```python
from build123d import *

# Parameters (mm, degrees)
F0_R     = 10.5
F0_R_2   = 6
F1_DEPTH = 15
F2_R     = 9
F2_R_2   = 6
F3_DEPTH = 10
F5_DEPTH = 4
F6_SIZE  = 0.5
F7_SIZE  = 0.5


with BuildPart() as f1:
    # F0 (on Top) → F1 (new body)
    with BuildSketch(Plane.XY):
        Circle(F0_R)
        Circle(F0_R_2, mode=Mode.SUBTRACT)
    extrude(amount=F1_DEPTH)

    # F2 (on face) → F3 (cut)
    with BuildSketch(Plane.XY.offset(15)):
        Circle(F2_R)
        Circle(F2_R_2, mode=Mode.SUBTRACT)
    extrude(amount=-F3_DEPTH, mode=Mode.SUBTRACT)

    # F4 (on face) → F5 (cut)
    with BuildSketch(Plane(origin=(0, 0, 0), x_dir=(1, 0, 0), z_dir=(0, 0, -1))):
        with BuildLine():
            Line((1.25, 8.25), (1.25, 13))
            Line((1.25, 13), (-1.25, 13))
            Line((-1.25, 13), (-1.25, 8.25))
            ThreePointArc((-1.25, 8.25), (-1.1767766953, 8.0732233047), (-1, 8))
            Line((-1, 8), (1, 8))
            ThreePointArc((1, 8), (1.1767766953, 8.0732233047), (1.25, 8.25))
        make_face()
        with BuildLine():
            Line((-6.5197095812, 5.2075317547), (-10.6333302492, 7.5825317547))
            Line((-10.6333302492, 7.5825317547), (-11.8833302492, 5.4174682453))
            Line((-11.8833302492, 5.4174682453), (-7.7697095812, 3.0424682453))
            ThreePointArc((-7.7697095812, 3.0424682453), (-7.5800048199, 3.0174931396), (-7.4282032303, 3.1339745962))
            Line((-7.4282032303, 3.1339745962), (-6.4282032303, 4.8660254038))
            ThreePointArc((-6.4282032303, 4.8660254038), (-6.4032281246, 5.0557301651), (-6.5197095812, 5.2075317547))
        make_face()
        with BuildLine():
            Line((-7.7697095812, -3.0424682453), (-11.8833302492, -5.4174682453))
            Line((-11.8833302492, -5.4174682453), (-10.6333302492, -7.5825317547))
            Line((-10.6333302492, -7.5825317547), (-6.5197095812, -5.2075317547))
            ThreePointArc((-6.5197095812, -5.2075317547), (-6.4032281246, -5.0557301651), (-6.4282032303, -4.8660254038))
            Line((-6.4282032303, -4.8660254038), (-7.4282032303, -3.1339745962))
            ThreePointArc((-7.4282032303, -3.1339745962), (-7.5800048199, -3.0174931396), (-7.7697095812, -3.0424682453))
        make_face()
        with BuildLine():
            Line((-1.25, -8.25), (-1.25, -13))
            Line((-1.25, -13), (1.25, -13))
            Line((1.25, -13), (1.25, -8.25))
            ThreePointArc((1.25, -8.25), (1.1767766953, -8.0732233047), (1, -8))
            Line((1, -8), (-1, -8))
            ThreePointArc((-1, -8), (-1.1767766953, -8.0732233047), (-1.25, -8.25))
        make_face()
        with BuildLine():
            Line((6.5197095812, -5.2075317547), (10.6333302492, -7.5825317547))
            Line((10.6333302492, -7.5825317547), (11.8833302492, -5.4174682453))
            Line((11.8833302492, -5.4174682453), (7.7697095812, -3.0424682453))
            ThreePointArc((7.7697095812, -3.0424682453), (7.5800048199, -3.0174931396), (7.4282032303, -3.1339745962))
            Line((7.4282032303, -3.1339745962), (6.4282032303, -4.8660254038))
            ThreePointArc((6.4282032303, -4.8660254038), (6.4032281246, -5.0557301651), (6.5197095812, -5.2075317547))
        make_face()
        with BuildLine():
            Line((7.7697095812, 3.0424682453), (11.8833302492, 5.4174682453))
            Line((11.8833302492, 5.4174682453), (10.6333302492, 7.5825317547))
            Line((10.6333302492, 7.5825317547), (6.5197095812, 5.2075317547))
            ThreePointArc((6.5197095812, 5.2075317547), (6.4032281246, 5.0557301651), (6.4282032303, 4.8660254038))
            Line((6.4282032303, 4.8660254038), (7.4282032303, 3.1339745962))
            ThreePointArc((7.4282032303, 3.1339745962), (7.5800048199, 3.0174931396), (7.7697095812, 3.0424682453))
        make_face()
    extrude(amount=-F5_DEPTH, mode=Mode.SUBTRACT)

    # F6
    f6_edges = [f1.edges().sort_by_distance(p)[0] for p in [
        (-5.25, -9.093267, 0),
        (5.25, -9.093267, 0),
        (10.286224, 2.107984, 0),
        (5.25, 9.093267, 0),
        (-5.25, 9.093267, 0),
        (-10.5, 0, 0),
    ]]
    chamfer(f6_edges, length=F6_SIZE)

    # F7
    f7_edges = [f1.edges().sort_by_distance(p)[0] for p in [
        (-10.5, 0, 15),
    ]]
    chamfer(f7_edges, length=F7_SIZE)


solid = f1.part
```
Geometry check sheet. Reference: the model listing, model coordinates, mm. A direction names the side the tool comes from. Coordinates: 2 decimals unless noted, no trailing zeros. Loops run counter-clockwise (first coordinate to the right, second up) from the corner with the lowest first, then second, coordinate; pieces in that order, holes last. Notation, with made-up numbers: (34, 44) -> (88, 44) arc R5 ccw to (88, 53) -> close; hole circle Ø7 at (79, -21). An arc over 180 degrees is marked (long way). Put each result on its own line as item: value.
1) Cross-section at A-A on y = 0. Record the boundary of the cut face in (x, z), plus the area to 3 significant figures.
Result set:
outline: (-10.5, 0.5) -> (-10, 0) -> (-6, 0) -> (-6, 5) -> (-9, 5) -> (-9, 15) -> (-10, 15) -> (-10.5, 14.5) -> close; (6, 0) -> (10, 0) -> (10.5, 0.5) -> (10.5, 14.5) -> (10, 15) -> (9, 15) -> (9, 5) -> (6, 5) -> close
area: 74.5 mm^2
2) Thickness scan on line 1 (Y direction, x = 0, z = 10.5); line 2 (Y direction, x = -6.75, z = 3.25); line 3 (Y direction, x = 0, z = 1.3). Record the ranges inside material, lowest first.
Result set:
line 1: y = -10.5 to -9, 9 to 10.5
line 2: y = -8.04 to -5.34, -4.31 to 4.31, 5.34 to 8.04
line 3: y = -8 to -6, 6 to 8
3) Cross-section at C-C on z = 7. Record the boundary of the cut face in (x, y), plus the area to 3 significant figures.
Result set:
outline: circle Ø21 at (0, 0); hole circle Ø18 at (0, 0)
area: 91.9 mm^2
4) Tool access check on faces 1 (the flat face through (-7.475, 5.759, 1.972)), 2 (the flat face through (1.25, -9, 2)), 3 (the flat face through (-1.25, 9, 2)). Record the directions out of +Z, -Z, +X, -X, +Y, -Y that give a thin tool (end or side, any length) a straight path to the whole face; none if there is none.
Result set:
face 1: -Z, -X
face 2: -Z, -Y
face 3: -Z, +Y
5) Cross-section at B-B on x = 0. Record the boundary of the cut face in (y, z).
Result set:
outline: (-10.5, 4) -> (-8, 4) -> (-8, 0) -> (-6, 0) -> (-6, 5) -> (-9, 5) -> (-9, 15) -> (-10, 15) -> (-10.5, 14.5) -> close; (6, 0) -> (8, 0) -> (8, 4) -> (10.5, 4) -> (10.5, 14.5) -> (10, 15) -> (9, 15) -> (9, 5) -> (6, 5) -> close
6) Gauge pin test, flat ends, axial feed: pin 1 Ø2 at (x, z) = (0, 2.5) entering from -Y; pin 2 Ø4 at (y, z) = (3.5, 3) entering from +X; pin 3 Ø1.2 at (x, y) = (-0.5, -10) entering from -Z; pin 4 Ø11 at (x, y) = (0, 0) entering from +Z. Record the tip position at first contact, or that the pin passes through.
Result set:
pin 1: stops at y = -8
pin 2: stops at x = 10.39
pin 3: stops at z = 4
pin 4: passes through
